Design review of the part built by this model. Coordinates are the model's own, in mm. Give positions to 0.01 mm unless a question says otherwise; leave off trailing zeros. Write each loop counter-clockwise with the first axis right and the second up, starting at its lowest first coordinate (ties: lowest second). Pieces come first, ordered by that corner, then holes.
```python
from build123d import *

# Parameters (mm, degrees)
F1_DEPTH = 2.54
F3_DEPTH = 12.7
F4_DEPTH = 2.54


# Not quite as in the source:
# - a feature names something its author has since deleted; it is built from what else it names


with BuildPart() as f1:
    # F0 (on Top) → F1 (new body)
    with BuildSketch(Plane.XY):
        with BuildLine():
            ThreePointArc((24.89835, -8.3058), (24.9076493597, -8.2833493597), (24.9301, -8.27405))
            Line((24.9301, -8.27405), (24.9301, 8.14705))
            ThreePointArc((24.9301, 8.14705), (24.9076493597, 8.1563493597), (24.89835, 8.1788))
            ThreePointArc((24.89835, 8.1788), (24.9301, 8.21055), (24.96185, 8.1788))
            Line((24.96185, 8.1788), (34.57575, 8.1788))
            ThreePointArc((34.57575, 8.1788), (34.5850493597, 8.2012506403), (34.6075, 8.21055))
            Line((34.6075, 8.21055), (34.6075, 9.36625))
            ThreePointArc((34.6075, 9.36625), (34.5850493597, 9.3755493597), (34.57575, 9.398))
            ThreePointArc((34.57575, 9.398), (34.5850493597, 9.4204506403), (34.6075, 9.42975))
            Line((34.6075, 9.42975), (34.6075, 26.38425))
            ThreePointArc((34.6075, 26.38425), (34.5850493597, 26.3935493597), (34.57575, 26.416))
            Line((34.57575, 26.416), (-34.57575, 26.416))
            ThreePointArc((-34.57575, 26.416), (-34.5850493597, 26.3935493597), (-34.6075, 26.38425))
            Line((-34.6075, 26.38425), (-34.6075, -26.38425))
            ThreePointArc((-34.6075, -26.38425), (-34.5850493597, -26.3935493597), (-34.57575, -26.416))
            Line((-34.57575, -26.416), (30.48635, -26.416))
            ThreePointArc((30.48635, -26.416), (30.5181, -26.38425), (30.54985, -26.416))
            Line((30.54985, -26.416), (34.57575, -26.416))
            ThreePointArc((34.57575, -26.416), (34.5850493597, -26.3935493597), (34.6075, -26.38425))
            Line((34.6075, -26.38425), (34.6075, -9.55675))
            ThreePointArc((34.6075, -9.55675), (34.5850493597, -9.5474506403), (34.57575, -9.525))
            ThreePointArc((34.57575, -9.525), (34.5850493597, -9.5025493597), (34.6075, -9.49325))
            Line((34.6075, -9.49325), (34.6075, -8.33755))
            ThreePointArc((34.6075, -8.33755), (34.5850493597, -8.3282506403), (34.57575, -8.3058))
            Line((34.57575, -8.3058), (24.96185, -8.3058))
            ThreePointArc((24.96185, -8.3058), (24.9301, -8.33755), (24.89835, -8.3058))
        make_face()
        with BuildLine():
            Line((-12.8397, -11.79195), (-12.8397, -18.61185))
            ThreePointArc((-12.8397, -18.61185), (-12.8172493597, -18.6211493597), (-12.80795, -18.6436))
            ThreePointArc((-12.80795, -18.6436), (-12.8397, -18.67535), (-12.87145, -18.6436))
            Line((-12.87145, -18.6436), (-22.68855, -18.6436))
            ThreePointArc((-22.68855, -18.6436), (-22.7203, -18.67535), (-22.75205, -18.6436))
            ThreePointArc((-22.75205, -18.6436), (-22.7427506403, -18.6211493597), (-22.7203, -18.61185))
            Line((-22.7203, -18.61185), (-22.7203, -11.79195))
            ThreePointArc((-22.7203, -11.79195), (-22.7427506403, -11.7826506403), (-22.75205, -11.7602))
            ThreePointArc((-22.75205, -11.7602), (-22.7203, -11.72845), (-22.68855, -11.7602))
            Line((-22.68855, -11.7602), (-12.87145, -11.7602))
            ThreePointArc((-12.87145, -11.7602), (-12.8397, -11.72845), (-12.80795, -11.7602))
            ThreePointArc((-12.80795, -11.7602), (-12.8172493597, -11.7826506403), (-12.8397, -11.79195))
        make_face(mode=Mode.SUBTRACT)
        with BuildLine():
            ThreePointArc((-12.21105, -24.6126), (-12.2017506403, -24.5901493597), (-12.1793, -24.58085))
            Line((-12.1793, -24.58085), (-12.1793, -20.91055))
            ThreePointArc((-12.1793, -20.91055), (-12.2017506403, -20.9012506403), (-12.21105, -20.8788))
            ThreePointArc((-12.21105, -20.8788), (-12.1793, -20.84705), (-12.14755, -20.8788))
            Line((-12.14755, -20.8788), (9.22655, -20.8788))
            ThreePointArc((9.22655, -20.8788), (9.2583, -20.84705), (9.29005, -20.8788))
            ThreePointArc((9.29005, -20.8788), (9.2807506403, -20.9012506403), (9.2583, -20.91055))
            Line((9.2583, -20.91055), (9.2583, -24.58085))
            ThreePointArc((9.2583, -24.58085), (9.2807506403, -24.5901493597), (9.29005, -24.6126))
            ThreePointArc((9.29005, -24.6126), (9.2583, -24.64435), (9.22655, -24.6126))
            Line((9.22655, -24.6126), (-12.14755, -24.6126))
            ThreePointArc((-12.14755, -24.6126), (-12.1793, -24.64435), (-12.21105, -24.6126))
        make_face(mode=Mode.SUBTRACT)
        with BuildLine():
            ThreePointArc((-7.4422, -15.875), (-8.3947, -16.8275), (-9.3472, -15.875))
            ThreePointArc((-9.3472, -15.875), (-8.3947, -14.9225), (-7.4422, -15.875))
        make_face(mode=Mode.SUBTRACT)
        with BuildLine():
            ThreePointArc((8.4328, -15.875), (7.4803, -16.8275), (6.5278, -15.875))
            ThreePointArc((6.5278, -15.875), (7.4803, -14.9225), (8.4328, -15.875))
        make_face(mode=Mode.SUBTRACT)
        with BuildLine():
            ThreePointArc((12.75715, -18.669), (12.7664493597, -18.6465493597), (12.7889, -18.63725))
            Line((12.7889, -18.63725), (12.7889, -10.82675))
            ThreePointArc((12.7889, -10.82675), (12.7664493597, -10.8174506403), (12.75715, -10.795))
            ThreePointArc((12.75715, -10.795), (12.7889, -10.76325), (12.82065, -10.795))
            Line((12.82065, -10.795), (18.90395, -10.795))
            ThreePointArc((18.90395, -10.795), (18.9357, -10.76325), (18.96745, -10.795))
            ThreePointArc((18.96745, -10.795), (18.9581506403, -10.8174506403), (18.9357, -10.82675))
            Line((18.9357, -10.82675), (18.9357, -18.63725))
            ThreePointArc((18.9357, -18.63725), (18.9581506403, -18.6465493597), (18.96745, -18.669))
            ThreePointArc((18.96745, -18.669), (18.9357, -18.70075), (18.90395, -18.669))
            Line((18.90395, -18.669), (12.82065, -18.669))
            ThreePointArc((12.82065, -18.669), (12.7889, -18.70075), (12.75715, -18.669))
        make_face(mode=Mode.SUBTRACT)
        with BuildLine():
            ThreePointArc((-15.367, 0), (-16.3195, -0.9525), (-17.272, 0))
            ThreePointArc((-17.272, 0), (-16.3195, 0.9525), (-15.367, 0))
        make_face(mode=Mode.SUBTRACT)
        with BuildLine():
            ThreePointArc((0.508, 0), (-0.4445, -0.9525), (-1.397, 0))
            ThreePointArc((-1.397, 0), (-0.4445, 0.9525), (0.508, 0))
        make_face(mode=Mode.SUBTRACT)
        with BuildLine():
            ThreePointArc((-28.067, 15.875), (-29.0195, 14.9225), (-29.972, 15.875))
            ThreePointArc((-29.972, 15.875), (-29.0195, 16.8275), (-28.067, 15.875))
        make_face(mode=Mode.SUBTRACT)
        with BuildLine():
            ThreePointArc((-7.4422, 15.875), (-8.3947, 14.9225), (-9.3472, 15.875))
            ThreePointArc((-9.3472, 15.875), (-8.3947, 16.8275), (-7.4422, 15.875))
        make_face(mode=Mode.SUBTRACT)
        with BuildLine():
            ThreePointArc((16.383, 0), (15.4305, -0.9525), (14.478, 0))
            ThreePointArc((14.478, 0), (15.4305, 0.9525), (16.383, 0))
        make_face(mode=Mode.SUBTRACT)
        with BuildLine():
            ThreePointArc((8.4328, 15.875), (7.4803, 14.9225), (6.5278, 15.875))
            ThreePointArc((6.5278, 15.875), (7.4803, 16.8275), (8.4328, 15.875))
        make_face(mode=Mode.SUBTRACT)
        with BuildLine():
            ThreePointArc((29.083, 15.875), (28.1305, 14.9225), (27.178, 15.875))
            ThreePointArc((27.178, 15.875), (28.1305, 16.8275), (29.083, 15.875))
        make_face(mode=Mode.SUBTRACT)
        with BuildLine():
            Line((12.7889, -10.82675), (12.7889, -18.63725))
            ThreePointArc((12.7889, -18.63725), (12.8113506403, -18.6465493597), (12.82065, -18.669))
            Line((12.82065, -18.669), (18.90395, -18.669))
            ThreePointArc((18.90395, -18.669), (18.9132493597, -18.6465493597), (18.9357, -18.63725))
            Line((18.9357, -18.63725), (18.9357, -10.82675))
            ThreePointArc((18.9357, -10.82675), (18.9132493597, -10.8174506403), (18.90395, -10.795))
            Line((18.90395, -10.795), (12.82065, -10.795))
            ThreePointArc((12.82065, -10.795), (12.8113506403, -10.8174506403), (12.7889, -10.82675))
        make_face()
        with BuildLine():
            Line((-12.1793, -20.91055), (-12.1793, -24.58085))
            ThreePointArc((-12.1793, -24.58085), (-12.1568493597, -24.5901493597), (-12.14755, -24.6126))
            Line((-12.14755, -24.6126), (9.22655, -24.6126))
            ThreePointArc((9.22655, -24.6126), (9.2358493597, -24.5901493597), (9.2583, -24.58085))
            Line((9.2583, -24.58085), (9.2583, -20.91055))
            ThreePointArc((9.2583, -20.91055), (9.2358493597, -20.9012506403), (9.22655, -20.8788))
            Line((9.22655, -20.8788), (-12.14755, -20.8788))
            ThreePointArc((-12.14755, -20.8788), (-12.1568493597, -20.9012506403), (-12.1793, -20.91055))
        make_face()
        with BuildLine():
            ThreePointArc((-12.87145, -18.6436), (-12.8621506403, -18.6211493597), (-12.8397, -18.61185))
            Line((-12.8397, -18.61185), (-12.8397, -11.79195))
            ThreePointArc((-12.8397, -11.79195), (-12.8621506403, -11.7826506403), (-12.87145, -11.7602))
            Line((-12.87145, -11.7602), (-22.68855, -11.7602))
            ThreePointArc((-22.68855, -11.7602), (-22.6978493597, -11.7826506403), (-22.7203, -11.79195))
            Line((-22.7203, -11.79195), (-22.7203, -18.61185))
            ThreePointArc((-22.7203, -18.61185), (-22.6978493597, -18.6211493597), (-22.68855, -18.6436))
            Line((-22.68855, -18.6436), (-12.87145, -18.6436))
        make_face()
    extrude(amount=F1_DEPTH)

    # F2 (on face) → F3 (join)
    with BuildSketch(Plane(origin=(0, 0, 0), x_dir=(1, 0, 0), z_dir=(0, 0, -1))):
        with BuildLine():
            Line((24.96185, -8.1788), (34.57575, -8.1788))
            Line((34.57575, -8.1788), (34.6075, 8.33755))
            ThreePointArc((34.6075, 8.33755), (34.5850493597, 8.3282506403), (34.57575, 8.3058))
            Line((34.57575, 8.3058), (24.96185, 8.3058))
            ThreePointArc((24.96185, 8.3058), (24.9076493597, 8.3282506403), (24.9301, 8.27405))
            Line((24.9301, 8.27405), (24.9301, -8.14705))
            ThreePointArc((24.9301, -8.14705), (24.9076493597, -8.2012506403), (24.96185, -8.1788))
        make_face()
    extrude(amount=F3_DEPTH)

    # F4 (add): a face of the model
    f4_faces = [f1.faces().sort_by_distance(p)[0] for p in [
        (29.7607313536, -0.0680465181, 0),
    ]]
    extrude(f4_faces, amount=F4_DEPTH)


solid = f1.part
```
(1) Consider section C-C, the plane x = -26. Give the boundary of the cut face in (y, z), then the cut area to 3 significant figures.
Resolved:
outline: (-26.42, 0) - (26.42, 0) - (26.42, 2.54) - (-26.42, 2.54) - close
area: 134 mm2
(2) Consider section D-D, the plane y = 22.5. Give the boundary of the cut face in (x, z), then the cut area to 3 significant figures.
Resolved:
outline: (-34.61, 0) - (34.61, 0) - (34.61, 2.54) - (-34.61, 2.54) - close
area: 176 mm2
(3) Mouldability with a two-part tool opening along X and no side actions: class faces 1 (the face through (-28.07, 15.92, 1.25)), 2 (the face through (24.93, 0, -6)), 3 (the face through (-7.639, -16.455, 1.252)) as pulls with the +X half, pulls with the -X half, needs draft (parallel to the pull), parting line crosses it, or undercut.
Resolved:
face 1: undercut
face 2: pulls with the -X half
face 3: undercut
(4) Clearance check with flat-ended pins moving along their axes: P1, Ø6.5, axis at y = 2, z = -8.5, coming from the -X side; P2, Ø1.1, axis at x = -16.32, y = 0, coming from the +Z side; P3, Ø1, axis at x = 10, y = -8, coming from the -Z side; P4, Ø3, axis at x = 29.5, z = -7, coming from the +Y side. State where each tip first meets the part, or that it passes through.
Resolved:
P1: stops at x = 24.93
P2: passes through
P3: stops at z = 0
P4: stops at y = 8.18
(5) Consider section B-B, the plane z = -2. Give the boundary of the cut face in (x, y).
Resolved:
outline: (24.93, -8.27) arc R0.03 ccw (long way) to (24.96, -8.31) - (34.58, -8.31) arc R0.03 ccw to (34.61, -8.34) - (34.58, 8.18) - (24.96, 8.18) arc R0.03 ccw (long way) to (24.93, 8.15) - close
(6) Consider section A-A, the plane y = 0. Give the boundary of the cut face in (x, z), then the cut area to 3 significant figures.
Resolved:
outline: (-34.61, 0) - (-17.27, 0) - (-17.27, 2.54) - (-34.61, 2.54) - close; (-15.37, 0) - (-1.4, 0) - (-1.4, 2.54) - (-15.37, 2.54) - close; (0.51, 0) - (14.48, 0) - (14.48, 2.54) - (0.51, 2.54) - close; (16.38, 0) - (24.93, 0) - (24.93, -12.7) - (34.59, -12.7) - (34.59, 2.54) - (16.38, 2.54) - close
area: 284 mm2
(7) To check wall thickness, follow L1, parallel to Z at x = 10, y = -9; L2, parallel to X at y = 2, z = -10.25. State the ranges of each line that lie inside material, in increasing order.
Resolved:
L1: z = 0 to 2.54
L2: x = 24.93 to 34.59
